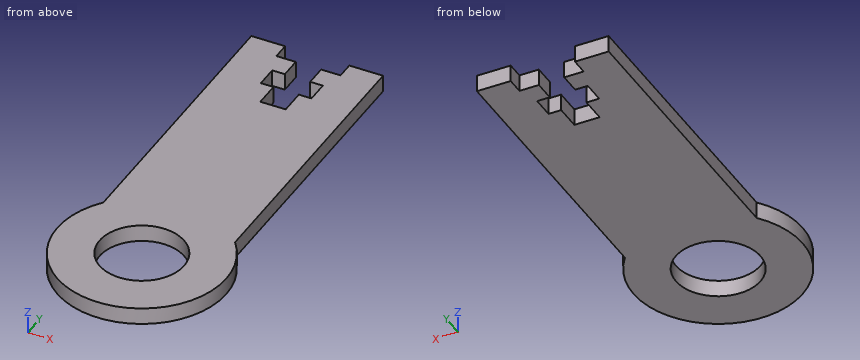
from build123d import *

# Parameters (mm, degrees)
SKETCH_1_R      = 5
EXTRUDE_1_DEPTH = 2


with BuildPart() as part:
    # 草图1 → 凸台-拉伸1 (new body)
    with BuildSketch(Plane.XY):
        with BuildLine():
            Line((0.753104923, 26.857612039), (3.053104923, 26.857612039))
            Line((3.053104923, 26.857612039), (3.053104923, 28.857612039))
            Line((3.053104923, 28.857612039), (7.053104923, 28.857612039))
            Line((7.053104923, 28.857612039), (7.053104923, -4.984592822))
            ThreePointArc((7.053104923, -4.984592822), (-0.746895077, -21.242387961), (-8.546895077, -4.984592822))
            Line((-8.546895077, -4.984592822), (-8.546895077, 28.857612039))
            Line((-8.546895077, 28.857612039), (-4.546895077, 28.857612039))
            Line((-4.546895077, 28.857612039), (-4.546895077, 26.857612039))
            Line((-4.546895077, 26.857612039), (-2.246895077, 26.857612039))
            Line((-2.246895077, 26.857612039), (-2.246895077, 24.357612039))
            Line((-2.246895077, 24.357612039), (-3.746895077, 24.357612039))
            Line((-3.746895077, 24.357612039), (-3.746895077, 21.757612039))
            Line((-3.746895077, 21.757612039), (-2.246895077, 21.757612039))
            Line((-2.246895077, 21.757612039), (-2.246895077, 18.757612039))
            Line((-2.246895077, 18.757612039), (0.753104923, 18.757612039))
            Line((0.753104923, 18.757612039), (0.753104923, 21.757612039))
            Line((0.753104923, 21.757612039), (2.253104923, 21.757612039))
            Line((2.253104923, 21.757612039), (2.253104923, 24.357612039))
            Line((2.253104923, 24.357612039), (0.753104923, 24.357612039))
            Line((0.753104923, 24.357612039), (0.753104923, 26.857612039))
        make_face()
        with Locations((-0.746895077, -11.242387961)):
            Circle(SKETCH_1_R, mode=Mode.SUBTRACT)
    extrude(amount=EXTRUDE_1_DEPTH)


solid = part.part
Check sheet for the modelled part. Datum: model origin and axes. Units: mm. Coordinates: 2 decimals unless noted, no trailing zeros. Write each loop counter-clockwise with the first axis right and the second up, starting at its lowest first coordinate (ties: lowest second). Pieces come first, ordered by that corner, then holes.
Item 1: Cross-section at A-A on y = 20. Record the boundary of the cut face in (x, z).
Numbers:
outline: (-8.55, 0) - (-2.25, 0) - (-2.25, 2) - (-8.55, 2) - close; (0.75, 0) - (7.05, 0) - (7.05, 2) - (0.75, 2) - close
Item 2: Depth check by flat-ended pin: pin 1 Ø1 at (y, z) = (23, 0.5) entering from -X; pin 2 Ø1 at (y, z) = (14, 1) entering from +X. Enter the tip coordinate at first touch or a pass-through.
Numbers:
pin 1: stops at x = -8.55
pin 2: stops at x = 7.05
Item 3: Scan lines: probe 1 along Y at (x, z) = (1.75, 0.6); probe 2 along X at (y, z) = (25, 0.5); probe 3 along Y at (x, z) = (-0.75, 0.15). Record each from-to range of solid material in increasing order.
Numbers:
probe 1: y = -20.93 to -15.57, -6.91 to 21.76, 24.36 to 26.86
probe 2: x = -8.55 to -2.25, 0.75 to 7.05
probe 3: y = -21.24 to -16.24, -6.24 to 18.76
Item 4: Cross-section at C-C on x = 0. Record the boundary of the cut face in (y, z), then the cut area to 3 significant figures.
Numbers:
outline: (-21.21, 0) - (-16.19, 0) - (-16.19, 2) - (-21.21, 2) - close; (-6.3, 0) - (18.76, 0) - (18.76, 2) - (-6.3, 2) - close
area: 60.2 mm2
Item 5: Cross-section at D-D on y = -0.5. Record the boundary of the cut face in (x, z), then the cut area to 3 significant figures.
Numbers:
outline: (-8.55, 0) - (7.05, 0) - (7.05, 2) - (-8.55, 2) - close
area: 31.2 mm2
Item 6: Cross-section at B-B on z = 1.55. Record the boundary of the cut face in (x, y), then the cut area to 3 significant figures.
Numbers:
outline: (-8.55, -4.98) arc R10 ccw (long way) to (7.05, -4.98) - (7.05, 28.86) - (3.05, 28.86) - (3.05, 26.86) - (0.75, 26.86) - (0.75, 24.36) - (2.25, 24.36) - (2.25, 21.76) - (0.75, 21.76) - (0.75, 18.76) - (-2.25, 18.76) - (-2.25, 21.76) - (-3.75, 21.76) - (-3.75, 24.36) - (-2.25, 24.36) - (-2.25, 26.86) - (-4.55, 26.86) - (-4.55, 28.86) - (-8.55, 28.86) - close; hole circle Ø10 at (-0.75, -11.24)
area: 676 mm2
